```python
from build123d import *

# Parameters (mm, degrees)
CHAMFER_1_SIZE  = 1.921
SKETCH_2_R      = 19.5
EXTRUDE_1_DEPTH = 30


with BuildPart() as part:
    # Эскиз1 → Повернуть1 (revolve)
    with BuildSketch(Plane.XY):
        Polygon((0, 6.5), (5, 6.5), (5, 15), (10, 15), (10, 13.079), (30, 13.079), (30, 19.5), (0, 19.5), align=None)
    revolve(axis=Axis((0, 0, 0), (1, 0, 0)))

    # Фаска1
    chamfer_1_edges = [part.edges().sort_by_distance(p)[0] for p in [
        (30, -13.079, 0),
    ]]
    chamfer(chamfer_1_edges, length=CHAMFER_1_SIZE)

    # Эскиз2 → Бобышка-Вытянуть1 (add)
    with BuildSketch(Plane(origin=(30, 0, 0), x_dir=(0, 0, -1), z_dir=(1, 0, 0))):
        Polygon((0, 23.094010768), (-20, 11.547005384), (-20, -11.547005384), (0, -23.094010768), (20, -11.547005384), (20, 11.547005384), align=None)
        Circle(SKETCH_2_R, mode=Mode.SUBTRACT)
    extrude(amount=-EXTRUDE_1_DEPTH)


solid = part.part
```
CAD build for the part. Positions are in the model's coordinates, mm. A direction names the side the tool comes from. Give positions to 0.01 mm unless a question says otherwise; leave off trailing zeros. Order: outer loops, then holes, each group sorted by start corner. A loop starts at its lowest first (then second) coordinate and runs counter-clockwise, first axis right, second up.
(1) Saw through at B-B, the plane x = 3.25. Give the cut face in (y, z).
(2) Flat gauge pins, fed straight in: pin 1 (1 mm diameter, centred on x = 8, z = 2.5, fed in from -Y); pin 2 (1 mm diameter, centred on y = 3.5, z = 8.5, fed in from +X); pin 3 (5 mm diameter, centred on x = 11, z = -12.5, fed in from -Y); pin 4 (1 mm diameter, centred on y = 13.5, z = 9.5, fed in from -X). Where does each tip first touch, or does it go through?
(3) Drill centre lines: L1, parallel to Z at x = 18, y = 0; L2, parallel to Z at x = 7.5, y = 0; L3, parallel to X at y = -12, z = 3. Where is each one in solid material? Low to high.
(4) Tool access for faces 4 (the flat face through (15, 0, 20)), 5 (the cylindrical face through (19.166, -2.835, -12.768)), 6 (the cylindrical face through (7.535, -14.985, 0.66)): list every direction of +Z, -Z, +X, -X, +Y, -Y with a clear straight run to the whole face (end or side of a thin tool).
(5) Saw through at A-A, the plane y = 0. Give the cut face in (x, z).
(6) Saw through at C-C, the plane x = 15.75. Give the cut face in (y, z).
(7) Mould opens along Y. For faces 1 (the conical face through (28.2, -1.72, 13.09)), 2 (the flat face through (30, -15, 5)), 3 (the flat face through (15.21, 17.24, -10.14)) say: released by +Y, released by -Y, zero draft, split by the parting line, or undercut.
(8) Saw through at D-D, the plane y = -17. Give the cut face in (x, z), then the cut area to 3 significant figures.
Results found:
1. outline: (-23.09, 0) - (-11.55, -20) - (11.55, -20) - (23.09, 0) - (11.55, 20) - (-11.55, 20) - close; hole circle Ø13 at (0, 0)
2. pin 1: stops at y = -21.94
2. pin 2: stops at x = 5
2. pin 3: stops at y = -17.32
2. pin 4: stops at x = 0
3. L1: z = -20 to -13.08, 13.08 to 20
3. L2: z = -20 to -15, 15 to 20
3. L3: x = 0 to 5
4. face 4: +Z, +X, -X, +Y, -Y
4. face 5: +X
4. face 6: none
5. outline: (0, -20) - (30, -20) - (30, -15) - (28.08, -13.08) - (10, -13.08) - (10, -15) - (5, -15) - (5, -6.5) - (0, -6.5) - close; (0, 6.5) - (5, 6.5) - (5, 15) - (10, 15) - (10, 13.08) - (28.08, 13.08) - (30, 15) - (30, 20) - (0, 20) - close
6. outline: (-23.09, 0) - (-11.55, -20) - (11.55, -20) - (23.09, 0) - (11.55, 20) - (-11.55, 20) - close; hole circle Ø26.16 at (0, 0)
7. face 1: undercut
7. face 2: zero draft
7. face 3: released by +Y
8. outline: (0, -10.56) - (30, -10.56) - (30, 10.56) - (0, 10.56) - close
8. area: 633 mm2
